```python
from build123d import *

# Parameters (mm, degrees)
SKETCH1_R           = 1.5
BOSS_EXTRUDE1_DEPTH = 3


with BuildPart() as part:
    # Sketch1 → Boss-Extrude1 (new body)
    with BuildSketch(Plane(origin=(0, 0, 0), x_dir=(1, 0, 0), z_dir=(0, 1, 0))):
        with BuildLine():
            Line((0, 50), (100, 50))
            Line((100, 50), (100, 70))
            Line((100, 70), (0, 70))
            ThreePointArc((0, 70), (-45.043425666, 53.582551304), (-68.958333333, 12.031137265))
            ThreePointArc((-68.958333333, 12.031137265), (-61.402498888, -14.934289299), (-48.958333333, 10.152910776))
            ThreePointArc((-48.958333333, 10.152910776), (-31.562275435, 38.779153799), (0, 50))
        make_face()
        with Locations(Location((-60, 0, 0), (0, 0, 270))):
            Circle(SKETCH1_R, mode=Mode.SUBTRACT)
    extrude(amount=BOSS_EXTRUDE1_DEPTH)


solid = part.part
```
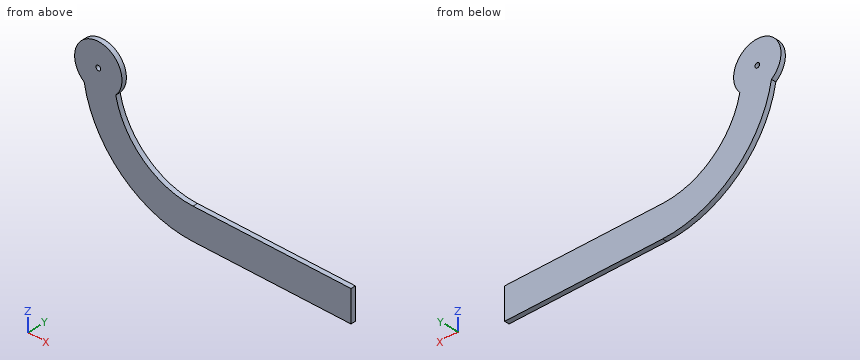
Verification items for the finished model (mm, model axes). Round coordinates to 2 decimals unless told otherwise and drop trailing zeros. Write each loop counter-clockwise with the first axis right and the second up, starting at its lowest first coordinate (ties: lowest second). Pieces come first, ordered by that corner, then holes.
1. Section check A-A on y = 1.9. Enter the section's corners in (x, z).
2. Scan lines: L1, parallel to X at y = 2.1, z = 0; L2, parallel to Z at x = 53, y = 0.2; L3, parallel to X at y = 0.5, z = -32.5. Record each from-to range of solid material in increasing order.
3. Section check B-B on x = 51.5. Enter the section's corners in (y, z), plus the area to 3 significant figures.
4. Gauge pin test, flat ends, axial feed: P1, Ø1, axis at y = 0.5, z = -35, coming from the -X side; P2, Ø1, axis at y = 0.5, z = -54.5, coming from the -X side; P3, Ø0.9, axis at x = 64, y = 1.5, coming from the +Z side. Record the tip position at first contact, or that the pin passes through.
5. Section check C-C on z = -44. Enter the section's corners in (x, y).
Answer:
1. outline: (-68.96, -12.03) arc R70 ccw to (0, -70) - (100, -70) - (100, -50) - (0, -50) arc R50 cw to (-48.96, -10.15) arc R15 ccw (long way) to start; hole circle Ø3 at (-60, 0)
2. L1: x = -75 to -61.5, -58.5 to -45
2. L2: z = -70 to -50
2. L3: x = -62 to -38
3. outline: (0, -70) - (3, -70) - (3, -50) - (0, -50) - close
3. area: 60.0 mm2
4. P1: stops at x = -60.91
4. P2: stops at x = -44.54
4. P3: stops at z = -50
5. outline: (-54.44, 0) - (-23.75, 0) - (-23.75, 3) - (-54.44, 3) - close
